Design review of the part shown in the three views and the two pictorial views. Dimensions are in mm from the part's minimum x, y and z. A direction names the side the tool comes from. Round coordinates to 2 decimals unless told otherwise and drop trailing zeros. Order: outer loops, then holes, each group sorted by start corner. A loop starts at its lowest first (then second) coordinate and runs counter-clockwise, first axis right, second up. Notation, with made-up numbers: (21.25, -12.5) -> (39.25, -12.5) arc R22 cw to (39.25, 3.5) -> close; hole circle Ø8 at (59.5, 74). An arc over 180 degrees is marked (long way). Put each result on its own line as item: value. Start each with the question number.
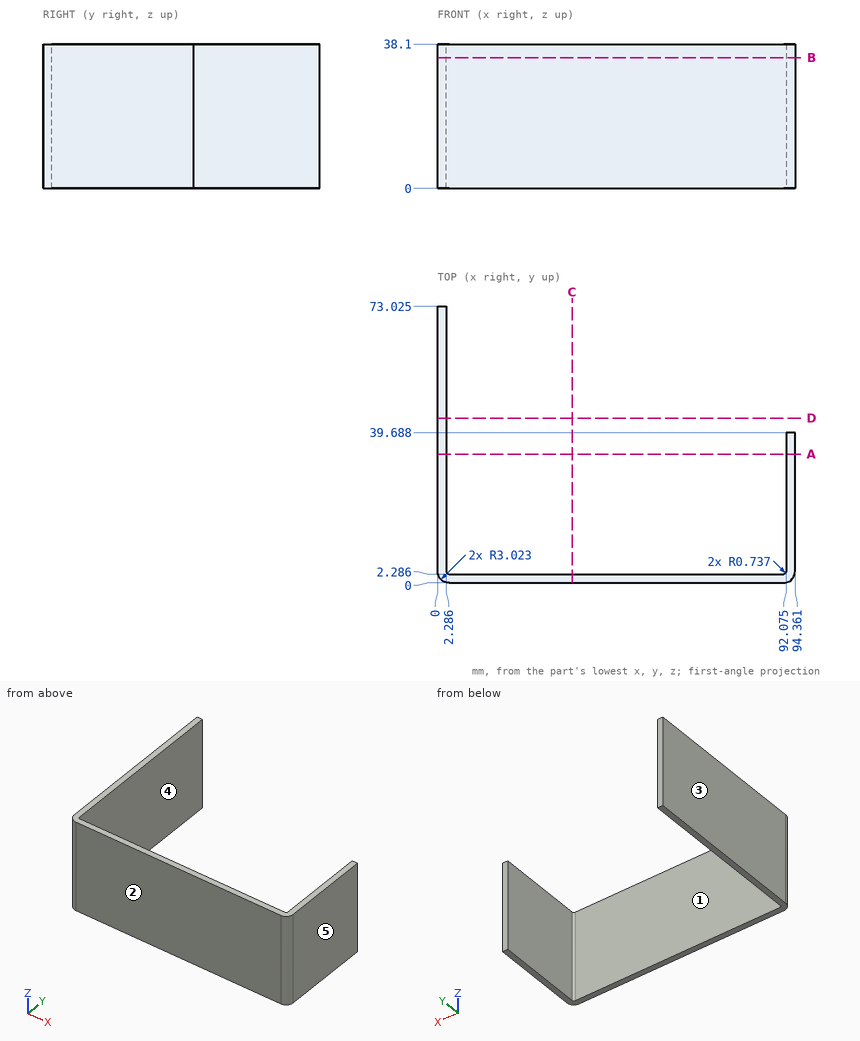
Q1. For the marked faces 4 and 5, list the 3-axis set-ups (+Z, -Z, +X, -X, +Y, -Y) from which the entire face can be reached by the end or side of a thin tool; tool diameter is ignored.
Q2. Clearance check with flat-ended pins moving along their axes: pin 1 Ø6 at (x, z) = (83.5, 32.5) entering from +Y; pin 2 Ø2.5 at (x, z) = (93, 14.5) entering from +Y. State where each tip first meets the part, or that it passes through.
Q3. Take a section at A-A on y = 34. Give the boundary of the cut face in (x, z) (1 decimal).
Q4. Wall thickness on probe 1 along X at (y, z) = (28.5, 16) (1 decimal); probe 2 along Y at (x, z) = (40.5, 8) (1 decimal): over which ranges is each line inside the solid? List them lowest first. Write a range as [from, to].
Q5. Take a section at C-C on x = 35.5. Give the boundary of the cut face in (y, z) (1 decimal).
Q6. Take a section at B-B on z = 34.5. Give the boundary of the cut face in (x, y) (1 decimal).
Q7. Draft analysis for pull direction X (two halves, no side actions). For the marked faces 1, 2 and 3, state which applies: +X half, -X half, draft (parallel to the pull), parting line (faces both ways), or undercut.
Calculated:
1. face 4: +Z, -Z, +Y
1. face 5: +Z, -Z, +X, +Y, -Y
2. pin 1: stops at y = 2.29
2. pin 2: stops at y = 39.69
3. outline: (0, 0) -> (2.3, 0) -> (2.3, 38.1) -> (0, 38.1) -> close; (92.1, 0) -> (94.4, 0) -> (94.4, 38.1) -> (92.1, 38.1) -> close
4. probe 1: x = [0, 2.3], [92.1, 94.4]
4. probe 2: y = [0, 2.3]
5. outline: (0, 0) -> (2.3, 0) -> (2.3, 38.1) -> (0, 38.1) -> close
6. outline: (0, 3) arc R3 ccw to (3, 0) -> (91.3, 0) arc R3 ccw to (94.4, 3) -> (94.4, 39.7) -> (92.1, 39.7) -> (92.1, 3) arc R0.7 cw to (91.3, 2.3) -> (3, 2.3) arc R0.7 cw to (2.3, 3) -> (2.3, 73) -> (0, 73) -> close
7. face 1: undercut
7. face 2: draft
7. face 3: -X half
